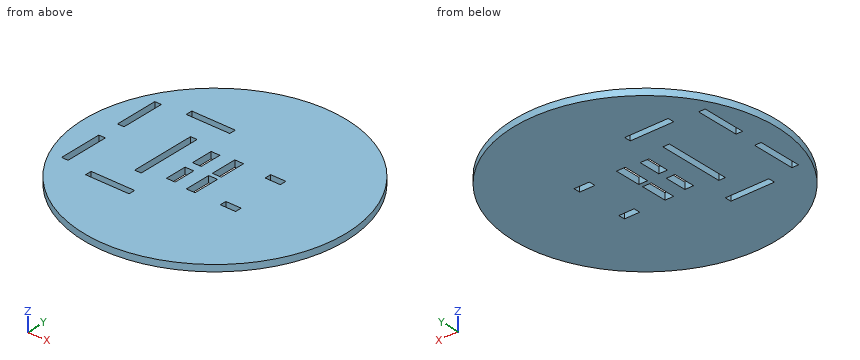
from build123d import *

# Parameters (mm, degrees)
SKETCH1_R           = 60
SKETCH1_W           = 20
SKETCH1_H           = 3
SKETCH1_W_2         = 3
SKETCH1_H_2         = 20
SKETCH1_H_3         = 30
SKETCH1_W_3         = 6.993462014
SKETCH1_W_4         = 4
SKETCH1_H_4         = 12
SKETCH1_H_5         = 10
BOSS_EXTRUDE1_DEPTH = 1.5


with BuildPart() as part:
    # Sketch1 → Boss-Extrude1 (new body, symmetric)
    with BuildSketch(Plane.XY):
        Circle(SKETCH1_R)
        with Locations((-25, -27)):
            Rectangle(SKETCH1_W, SKETCH1_H, mode=Mode.SUBTRACT)
        with Locations((-47.5, 15)):
            Rectangle(SKETCH1_W_2, SKETCH1_H_2, mode=Mode.SUBTRACT)
        with Locations((-47.5, -15)):
            Rectangle(SKETCH1_W_2, SKETCH1_H_2, mode=Mode.SUBTRACT)
        with Locations((-22.5, 0)):
            Rectangle(SKETCH1_W_2, SKETCH1_H_3, mode=Mode.SUBTRACT)
        with Locations((-25, 27)):
            Rectangle(SKETCH1_W, SKETCH1_H, mode=Mode.SUBTRACT)
        with Locations((17.516157806, -12)):
            Rectangle(SKETCH1_W_3, SKETCH1_H, mode=Mode.SUBTRACT)
        with Locations((17.516157806, 12)):
            Rectangle(SKETCH1_W_3, SKETCH1_H, mode=Mode.SUBTRACT)
        with Locations((0, 7)):
            Rectangle(SKETCH1_W_4, SKETCH1_H_4, mode=Mode.SUBTRACT)
        with Locations((0, -7)):
            Rectangle(SKETCH1_W_4, SKETCH1_H_4, mode=Mode.SUBTRACT)
        with Locations((-10, 7)):
            Rectangle(SKETCH1_W_4, SKETCH1_H_5, mode=Mode.SUBTRACT)
        with Locations((-10, -7)):
            Rectangle(SKETCH1_W_4, SKETCH1_H_5, mode=Mode.SUBTRACT)
    extrude(amount=BOSS_EXTRUDE1_DEPTH, both=True)


solid = part.part
Check sheet for the modelled part. Datum: model origin and axes. Units: mm. Give positions to 0.01 mm unless a question says otherwise; leave off trailing zeros. Loops run counter-clockwise (first coordinate to the right, second up) from the corner with the lowest first, then second, coordinate; pieces in that order, holes last. Notation, with made-up numbers: M 19.5,-11.5 L 45.5,-11.5 A21 cw 45.5,-4.5 Z; hole C -3.75,47 d4. An arc over 180 degrees is marked long. Use a Markdown table: item, result. Add a question column.
Q1. Sectioned sample at B-B, the plane y = 9. Record the cut outline in (x, z).
Q2. Sectioned sample at A-A, the plane x = 0. Record the cut outline in (y, z).
Q3. Sectioned sample at D-D, the plane y = -36. Record the cut outline in (x, z).
Q4. Go/stop test with flat-tipped pins: pin 1 (1.5 mm diameter, centred on y = -18, z = 0, fed in from +X); pin 2 (0.9 mm diameter, centred on y = 7, z = -0.5, fed in from +X); pin 3 (0.9 mm diameter, centred on y = -13, z = -0.5, fed in from -X). Record where each tip stops, or that it passes through.
Q5. Scan lines: line 1 along Y through (x, z) = (1.5, -0.1); line 2 along Y through (x, z) = (15, -0.5); line 3 along Y through (x, z) = (-22, -0.75). Record each from-to range of solid material in increasing order. Write a range as [from, to].
Q6. Sectioned sample at C-C, the plane z = 0.9. Give the number of separate pieces and of enclosed holes in the cut face, then the cut area to 3 significant figures.
Verdict:
| question | item | result |
|---|---|---|
| 1 | outline | M -59.32,-1.5 L -49,-1.5 L -49,1.5 L -59.32,1.5 Z; M -46,-1.5 L -24,-1.5 L -24,1.5 L -46,1.5 Z; M -21,-1.5 L -12,-1.5 L -12,1.5 L -21,1.5 Z; M -8,-1.5 L -2,-1.5 L -2,1.5 L -8,1.5 Z; M 2,-1.5 L 59.32,-1.5 L 59.32,1.5 L 2,1.5 Z |
| 2 | outline | M -60,-1.5 L -13,-1.5 L -13,1.5 L -60,1.5 Z; M -1,-1.5 L 1,-1.5 L 1,1.5 L -1,1.5 Z; M 13,-1.5 L 60,-1.5 L 60,1.5 L 13,1.5 Z |
| 3 | outline | M -48,-1.5 L 48,-1.5 L 48,1.5 L -48,1.5 Z |
| 4 | pin 1 | x = 57.47 |
| 4 | pin 2 | x = 59.64 |
| 4 | pin 3 | x = -58.67 |
| 5 | line 1 | [-59.98, -13], [-1, 1], [13, 59.98] |
| 5 | line 2 | [-58.09, -13.5], [-10.5, 10.5], [13.5, 58.09] |
| 5 | line 3 | [-55.82, -28.5], [-25.5, -15], [15, 25.5], [28.5, 55.82] |
| 6 | separate pieces | 1 |
| 6 | enclosed holes | 11 |
| 6 | area | 10,800 mm^2 |
